Read the model definition and answer for the solid it produces. Units are mm, in the model's axes. A direction names the side the tool comes from. Coordinates: 2 decimals unless noted, no trailing zeros. Answer as a JSON object with one key per item and string values. Group by question number.
1) Section A-A on x = 0 is taken. Count the separate pieces of the cut face and the enclosed holes in it, and give its area (3 significant figures).
2) A tool of negligible diameter and unlimited length cuts with its end or side. For faces 3 (the cylindrical face through (-3.905, 1.479, -0.867)), 4 (the flat face through (-9.475, 3.014, 3.511)), from which of +Z, -Z, +X, -X, +Y, -Y can it reach the whole face along a straight path? Write none if from no direction.
3) Given pin 1 (1.5 mm diameter, centred on x = -24, y = 3, fed in from +Z); pin 2 (2 mm diameter, centred on x = -8.5, z = 5, fed in from +Y); pin 3 (3 mm diameter, centred on x = 24.51, z = -4.91, fed in from -Y); pin 4 (7 mm diameter, centred on x = -21.65, z = 12.5, fed in from +Y), each flat-ended and moving along its own axis, determine where each tip first touches the part or whether it passes through.
4) Consider L1, parallel to X at y = 1.65, z = -0.5; L2, parallel to Z at x = -8.5, y = 3.7; L3, parallel to X at y = 0.95, z = 5. Determine where each line is inside the solid, lowest interval first.
5) Determine the mould class of faces 1 (the flat face through (-7, 0, 0)), 2 (the flat face through (1, 2, -10)) for opening direction X: released by +X, released by -X, zero draft, split by the parting line, or undercut.
from build123d import *

# Parameters (mm, degrees)
SKETCH_1_R          = 32
SKETCH_1_R_2        = 4
SKETCH_1_R_3        = 3
EXTRUDE_1_DEPTH     = 4
FILLET_1_R          = 2
SKETCH_2_R          = 1.1
CUT_EXTRUDE_1_DEPTH = 46.431266766
SKETCH_3_R          = 1.6
CUT_EXTRUDE_2_DEPTH = 46.431266766
CUT_EXTRUDE_3_DEPTH = 2
CHAMFER_1_SIZE      = 1
SKETCH_5_R          = 0.9
CUT_EXTRUDE_4_DEPTH = 46.431266766


with BuildPart() as part:
    # Эскиз1 → Бобышка-Вытянуть1 (new body)
    with BuildSketch(Plane(origin=(0, 0, 0), x_dir=(1, 0, 0), z_dir=(0, 1, 0))):
        with Locations(Location((0, 0, 0), (0, 0, 270))):
            Circle(SKETCH_1_R)
        with Locations(Location((0, 0, 0), (0, 0, 270))):
            Circle(SKETCH_1_R_2, mode=Mode.SUBTRACT)
        with Locations(Location((0, 25, 0), (0, 0, 270))):
            Circle(SKETCH_1_R_3, mode=Mode.SUBTRACT)
        with Locations(Location((21.650635095, -12.5, 0), (0, 0, 270))):
            Circle(SKETCH_1_R_3, mode=Mode.SUBTRACT)
        with Locations(Location((-21.650635095, -12.5, 0), (0, 0, 270))):
            Circle(SKETCH_1_R_3, mode=Mode.SUBTRACT)
    extrude(amount=EXTRUDE_1_DEPTH)

    # Скругление1
    fillet_1_edges = [part.edges().sort_by_distance(p)[0] for p in [
        (0, 4, -32),
    ]]
    fillet(fillet_1_edges, radius=FILLET_1_R)

    # Эскиз2 → Вырез-Вытянуть1 (cut, through all)
    with BuildSketch(Plane(origin=(0, 4, 0), x_dir=(1, 0, 0), z_dir=(0, 1, 0))):
        with Locations(Location((0, 9, 0), (0, 0, 270))):
            Circle(SKETCH_2_R)
        with Locations(Location((7.794228634, -4.5, 0), (0, 0, 270))):
            Circle(SKETCH_2_R)
        with Locations(Location((-7.794228634, -4.5, 0), (0, 0, 270))):
            Circle(SKETCH_2_R)
    extrude(amount=-CUT_EXTRUDE_1_DEPTH, mode=Mode.SUBTRACT)

    # Эскиз3 → Вырез-Вытянуть2 (cut, through all)
    with BuildSketch(Plane.XZ):
        with Locations(Location((0, 14, 0), (0, 0, 270))):
            Circle(SKETCH_3_R)
        with Locations(Location((14, 0, 0), (0, 0, 270))):
            Circle(SKETCH_3_R)
        with Locations(Location((0, -14, 0), (0, 0, 270))):
            Circle(SKETCH_3_R)
        with Locations(Location((-14, 0, 0), (0, 0, 270))):
            Circle(SKETCH_3_R)
    extrude(amount=-CUT_EXTRUDE_2_DEPTH, mode=Mode.SUBTRACT)

    # Эскиз4 → Вырез-Вытянуть3 (cut)
    with BuildSketch(Plane(origin=(0, 4, 0), x_dir=(1, 0, 0), z_dir=(0, 1, 0))):
        Polygon((5.542562584, -4.5), (6.668395609, -6.45), (8.920061659, -6.45), (10.045894684, -4.5), (8.920061659, -2.55), (6.668395609, -2.55), align=None)
        Polygon((1.125833025, 7.05), (2.25166605, 9), (1.125833025, 10.95), (-1.125833025, 10.95), (-2.25166605, 9), (-1.125833025, 7.05), align=None)
        Polygon((-6.668395609, -2.55), (-8.920061659, -2.55), (-10.045894684, -4.5), (-8.920061659, -6.45), (-6.668395609, -6.45), (-5.542562584, -4.5), align=None)
    extrude(amount=-CUT_EXTRUDE_3_DEPTH, mode=Mode.SUBTRACT)

    # Фаска1
    chamfer_1_edges = [part.edges().sort_by_distance(p)[0] for p in [
        (21.650635095, 4, 9.5),
        (-21.650635095, 4, 9.5),
        (0, 4, -4),
        (0, 4, -28),
    ]]
    chamfer(chamfer_1_edges, length=CHAMFER_1_SIZE)

    # Эскиз5 → Вырез-Вытянуть4 (cut, through all)
    with BuildSketch(Plane(origin=(0, 4, 0), x_dir=(1, 0, 0), z_dir=(0, 1, 0))):
        with Locations(Location((-8, -23.685438565, 0), (0, 0, 270))):
            Circle(SKETCH_5_R)
        with Locations(Location((8, -23.685438565, 0), (0, 0, 270))):
            Circle(SKETCH_5_R)
        with Locations(Location((-16.512191497, 18.770922513, 0), (0, 0, 270))):
            Circle(SKETCH_5_R)
        with Locations(Location((-24.512191497, 4.914516052, 0), (0, 0, 270))):
            Circle(SKETCH_5_R)
        with Locations(Location((24.512191497, 4.914516052, 0), (0, 0, 270))):
            Circle(SKETCH_5_R)
        with Locations(Location((16.512191497, 18.770922513, 0), (0, 0, 270))):
            Circle(SKETCH_5_R)
    extrude(amount=-CUT_EXTRUDE_4_DEPTH, mode=Mode.SUBTRACT)


solid = part.part
Worked answers:
{
 "1": {"separate pieces": "6", "enclosed holes": "0", "area": "158 mm²"},
 "2": {"face 3": "+Y, -Y", "face 4": "+Y"},
 "3": {"pin 1": "stops at z = 21.74", "pin 2": "stops at y = 2", "pin 3": "stops at y = 0", "pin 4": "stops at y = 3.5"},
 "4": {"L1": "x = -32 to -15.52, -12.48 to -3.97, 3.97 to 12.48, 15.52 to 32", "L2": "z = -29.87 to 2.55, 6.45 to 22.94, 24.43 to 29.87", "L3": "x = -31.61 to -8.77, -6.81 to 6.81, 8.77 to 31.61"},
 "5": {"face 1": "zero draft", "face 2": "undercut"}
}
